Input: part model. Units: mm. Frame: model coordinates. Give positions to 0.01 mm unless a question says otherwise; leave off trailing zeros. Loops run counter-clockwise (first coordinate to the right, second up) from the corner with the lowest first, then second, coordinate; pieces in that order, holes last. Notation, with made-up numbers: M -16.75,51 L 42.25,51 A15 cw 42.25,55 Z; hole C -39.5,61.25 d1. An arc over 180 degrees is marked long. Return JSON: item names as keys, results as strings. Group by question number.
```python
from build123d import *

# Parameters (mm, degrees)
F1_DEPTH = 50.8
F3_DEPTH = 44.451
F4_DEPTH = 25.4


# Not quite as in the source:
# - ends of sketch curves that miss each other by under 0.0002 mm in the source are joined


with BuildPart() as f1:
    # F0 (on Front) → F1 (new body, symmetric)
    with BuildSketch(Plane.XZ):
        Polygon((-347.7068640215, -34.8248227949), (-347.7068640215, -79.2748227949), (367.1742644244, -79.272822397), (408.7938746644, -44.3498227949), (414.2931359785, -34.8248227949), align=None)
    extrude(amount=F1_DEPTH, both=True)

    # F2 (on face) → F3 (cut, through all)
    with BuildSketch(Plane.XY.offset(-34.8248227949)):
        with BuildLine():
            ThreePointArc((-304.0188640215, -12.7), (-296.9068640215, -19.812), (-289.7948640215, -12.7))
            Line((-289.7948640215, -12.7), (-289.7948640215, 12.7))
            ThreePointArc((-289.7948640215, 12.7), (-296.9068640215, 19.812), (-304.0188640215, 12.7))
            Line((-304.0188640215, 12.7), (-304.0188640215, -12.7))
        make_face()
        with BuildLine():
            ThreePointArc((-151.6188640215, -12.7), (-144.5068640215, -19.812), (-137.3948640215, -12.7))
            Line((-137.3948640215, -12.7), (-137.3948640215, 12.7))
            ThreePointArc((-137.3948640215, 12.7), (-144.5068640215, 19.812), (-151.6188640215, 12.7))
            Line((-151.6188640215, 12.7), (-151.6188640215, -12.7))
        make_face()
        with BuildLine():
            ThreePointArc((0.7811359785, -12.7), (7.8931359785, -19.812), (15.0051359785, -12.7))
            Line((15.0051359785, -12.7), (15.0051359785, 12.7))
            ThreePointArc((15.0051359785, 12.7), (7.8931359785, 19.812), (0.7811359785, 12.7))
            Line((0.7811359785, 12.7), (0.7811359785, -12.7))
        make_face()
        with BuildLine():
            ThreePointArc((153.1811359785, -12.7), (160.2931359785, -19.812), (167.4051359785, -12.7))
            Line((167.4051359785, -12.7), (167.4051359785, 12.7))
            ThreePointArc((167.4051359785, 12.7), (160.2931359785, 19.812), (153.1811359785, 12.7))
            Line((153.1811359785, 12.7), (153.1811359785, -12.7))
        make_face()
        with BuildLine():
            ThreePointArc((305.5811359785, -12.7), (312.6931359785, -19.812), (319.8051359785, -12.7))
            Line((319.8051359785, -12.7), (319.8051359785, 12.7))
            ThreePointArc((319.8051359785, 12.7), (312.6931359785, 19.812), (305.5811359785, 12.7))
            Line((305.5811359785, 12.7), (305.5811359785, -12.7))
        make_face()
    extrude(amount=-F3_DEPTH, mode=Mode.SUBTRACT)

    # F2 (on face) → F4 (cut)
    with BuildSketch(Plane.XY.offset(-34.8248227949)):
        with BuildLine():
            ThreePointArc((-283.4448517417, 12.7), (-296.9068640215, 26.1620122798), (-310.3688763013, 12.7))
            Line((-310.3688763013, 12.7), (-310.3688640215, -12.7))
            ThreePointArc((-310.3688640215, -12.7), (-296.9068640215, -26.162), (-283.4448640215, -12.7))
            Line((-283.4448640215, -12.7), (-283.4448517417, 12.7))
        make_face()
        with BuildLine():
            Line((-289.7948640215, 12.7), (-289.7948640215, -12.7))
            ThreePointArc((-289.7948640215, -12.7), (-296.9068640215, -19.812), (-304.0188640215, -12.7))
            Line((-304.0188640215, -12.7), (-304.0188640215, 12.7))
            ThreePointArc((-304.0188640215, 12.7), (-296.9068640215, 19.812), (-289.7948640215, 12.7))
        make_face(mode=Mode.SUBTRACT)
        with BuildLine():
            Line((-157.9688640215, 12.7), (-157.9688640215, -12.7))
            ThreePointArc((-157.9688640215, -12.7), (-144.5068640215, -26.162), (-131.0448640215, -12.7))
            Line((-131.0448640215, -12.7), (-131.0448516369, 12.7))
            ThreePointArc((-131.0448516369, 12.7), (-144.5068640215, 26.1620122798), (-157.9688640215, 12.7))
        make_face()
        with BuildLine():
            Line((-137.3948640215, 12.7), (-137.3948640215, -12.7))
            ThreePointArc((-137.3948640215, -12.7), (-144.5068640215, -19.812), (-151.6188640215, -12.7))
            Line((-151.6188640215, -12.7), (-151.6188640215, 12.7))
            ThreePointArc((-151.6188640215, 12.7), (-144.5068640215, 19.812), (-137.3948640215, 12.7))
        make_face(mode=Mode.SUBTRACT)
        with BuildLine():
            Line((-5.5688640215, 12.7), (-5.5688640215, -12.7))
            ThreePointArc((-5.5688640215, -12.7), (7.8931359785, -26.162), (21.3551359785, -12.7))
            Line((21.3551359785, -12.7), (21.3551483631, 12.7))
            ThreePointArc((21.3551483631, 12.7), (7.8931359785, 26.1620122798), (-5.5688640215, 12.7))
        make_face()
        with BuildLine():
            Line((15.0051359785, 12.7), (15.0051359785, -12.7))
            ThreePointArc((15.0051359785, -12.7), (7.8931359785, -19.812), (0.7811359785, -12.7))
            Line((0.7811359785, -12.7), (0.7811359785, 12.7))
            ThreePointArc((0.7811359785, 12.7), (7.8931359785, 19.812), (15.0051359785, 12.7))
        make_face(mode=Mode.SUBTRACT)
        with BuildLine():
            Line((146.8311359785, 12.7), (146.8311359785, -12.7))
            ThreePointArc((146.8311359785, -12.7), (160.2931359785, -26.162), (173.7551359785, -12.7))
            Line((173.7551359785, -12.7), (173.7551483631, 12.7))
            ThreePointArc((173.7551483631, 12.7), (160.2931359785, 26.1620122798), (146.8311359785, 12.7))
        make_face()
        with BuildLine():
            Line((167.4051359785, 12.7), (167.4051359785, -12.7))
            ThreePointArc((167.4051359785, -12.7), (160.2931359785, -19.812), (153.1811359785, -12.7))
            Line((153.1811359785, -12.7), (153.1811359785, 12.7))
            ThreePointArc((153.1811359785, 12.7), (160.2931359785, 19.812), (167.4051359785, 12.7))
        make_face(mode=Mode.SUBTRACT)
        with BuildLine():
            Line((299.2311359785, 12.7), (299.2311359785, -12.7))
            ThreePointArc((299.2311359785, -12.7), (312.6931359785, -26.162), (326.1551359785, -12.7))
            Line((326.1551359785, -12.7), (326.1551483631, 12.7))
            ThreePointArc((326.1551483631, 12.7), (312.6931359785, 26.1620122798), (299.2311359785, 12.7))
        make_face()
        with BuildLine():
            Line((319.8051359785, 12.7), (319.8051359785, -12.7))
            ThreePointArc((319.8051359785, -12.7), (312.6931359785, -19.812), (305.5811359785, -12.7))
            Line((305.5811359785, -12.7), (305.5811359785, 12.7))
            ThreePointArc((305.5811359785, 12.7), (312.6931359785, 19.812), (319.8051359785, 12.7))
        make_face(mode=Mode.SUBTRACT)
    extrude(amount=-F4_DEPTH, mode=Mode.SUBTRACT)


solid = f1.part
```
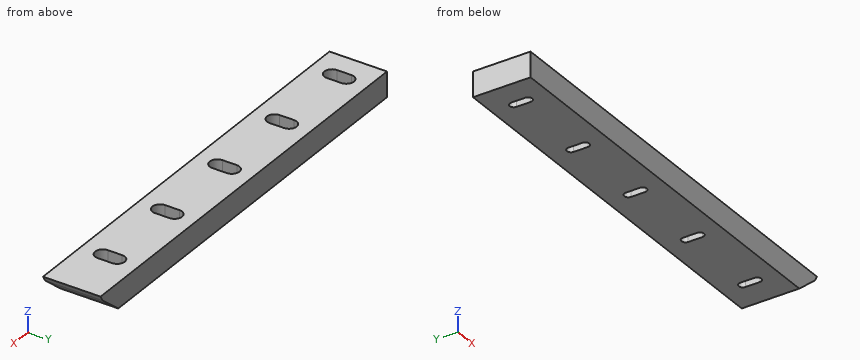
Item 1: First-contact query: pin 1 Ø6 at (y, z) = (-23.5, -52) entering from +X; pin 2 Ø13.5 at (x, y) = (164, -5) entering from +Z; pin 3 Ø15 at (y, z) = (-5, -74) entering from +X. Flat tips, straight axial feed; report the tip coordinate or a pass-through.
Item 2: Material intervals for line 1 (X direction, y = -22, z = -47.5); line 2 (X direction, y = -1.5, z = -63.5); line 3 (Y direction, x = 3.5, z = -38) (3 decimals), sorted ascending. Write a range as from..to.
Item 3: Section B-B, the plane y = 37. Return loops of the section in (x, z).
Item 4: Section A-A, the plane z = -71.5. Return loops of the section in (x, y), then the cut area to 3 significant figures.
Answer below:
{
 "1": {"pin 1": "x = 403.25", "pin 2": "z = -60.22", "pin 3": "x = 382.4"},
 "2": {"line 1": "-347.71..-306.64, -287.17..-154.24, -134.77..-1.84, 17.63..150.56, 170.03..302.96, 322.43..405.04", "line 2": "-347.71..-304.02, -289.79..-151.62, -137.39..0.78, 15.01..153.18, 167.41..305.58, 319.81..385.97", "line 3": "-50.8..-25.425, 25.425..50.8"},
 "3": {"outline": "M -347.71,-79.27 L 367.17,-79.27 L 408.79,-44.35 L 414.29,-34.82 L -347.71,-34.82 Z"},
 "4": {"outline": "M -347.71,-50.8 L 376.44,-50.8 L 376.44,50.8 L -347.71,50.8 Z; hole M -304.02,-12.7 A7.11 ccw -289.79,-12.7 L -289.79,12.7 A7.11 ccw -304.02,12.7 Z; hole M -151.62,-12.7 A7.11 ccw -137.39,-12.7 L -137.39,12.7 A7.11 ccw -151.62,12.7 Z; hole M 0.78,-12.7 A7.11 ccw 15.01,-12.7 L 15.01,12.7 A7.11 ccw 0.78,12.7 Z; hole M 153.18,-12.7 A7.11 ccw 167.41,-12.7 L 167.41,12.7 A7.11 ccw 153.18,12.7 Z; hole M 305.58,-12.7 A7.11 ccw 319.81,-12.7 L 319.81,12.7 A7.11 ccw 305.58,12.7 Z", "area": "71,000 mm^2"}
}
